```python
from build123d import *

# Parameters (mm, degrees)
SKETCH1_R           = 2
BOSS_EXTRUDE1_DEPTH = 16.85


with BuildPart() as part:
    # Sketch1 → Boss-Extrude1 (new body)
    # profile 1 of 4: a face of its own
    with BuildSketch(Plane(origin=(0, 0, 0), x_dir=(1, 0, 0), z_dir=(0, 1, 0))):
        Polygon((-24.645, 9), (-29.841152423, 0), (-24.841152423, 0), (0, 0), (0, 9), align=None)
        with Locations(Location((-14.92, 4.5, 0), (0, 0, 270))):
            Circle(SKETCH1_R, mode=Mode.SUBTRACT)
    # profile 2 of 4: a face of its own
    with BuildSketch(Plane(origin=(0, 0, 0), x_dir=(1, 0, 0), z_dir=(0, 1, 0))):
        Polygon((0, 9), (0, 0), (24.841152423, 0), (29.841152423, 0), (24.645, 9), align=None)
        with Locations(Location((14.92, 4.5, 0), (0, 0, 270))):
            Circle(SKETCH1_R, mode=Mode.SUBTRACT)
    # profile 3 of 4: a face of its own
    with BuildSketch(Plane(origin=(0, 0, 0), x_dir=(1, 0, 0), z_dir=(0, 1, 0))):
        with BuildLine():
            Line((-24.841152423, 0), (-29.841152423, 0))
            Line((-29.841152423, 0), (-42.542858345, -22))
            Line((-42.542858345, -22), (-38.697558883, -22))
            ThreePointArc((-38.697558883, -22), (-37.697558883, -21.732050808), (-36.965508076, -21))
            Line((-36.965508076, -21), (-24.841152423, 0))
        make_face()
    # profile 4 of 4: a face of its own
    with BuildSketch(Plane(origin=(0, 0, 0), x_dir=(1, 0, 0), z_dir=(0, 1, 0))):
        with BuildLine():
            Line((29.841152423, 0), (24.841152423, 0))
            Line((24.841152423, 0), (36.965508076, -21))
            ThreePointArc((36.965508076, -21), (37.697558883, -21.732050808), (38.697558883, -22))
            Line((38.697558883, -22), (42.542858345, -22))
            Line((42.542858345, -22), (29.841152423, 0))
        make_face()
    extrude(amount=BOSS_EXTRUDE1_DEPTH)


solid = part.part
```
Design review of the part built by this model. Coordinates are the model's own, in mm. A direction names the side the tool comes from. Round coordinates to 2 decimals unless told otherwise and drop trailing zeros. Order: outer loops, then holes, each group sorted by start corner. A loop starts at its lowest first (then second) coordinate and runs counter-clockwise, first axis right, second up. Notation, with made-up numbers: (41, 42.25) - (76, 42.25) arc R37 cw to (76, 78.25) - close; hole circle Ø1 at (57.5, 81). An arc over 180 degrees is marked (long way). One line per question, with ' | ' between items.
Item 1: Draft analysis for pull direction Z (two halves, no side actions). For faces 1 (the face through (0, 8, -9)), 2 (the face through (-16.872, 8.307, -4.934)), 3 (the face through (0, 0, -2)), 4 (the face through (0, 8, 0)), state which applies: +Z half, -Z half, draft (parallel to the pull), parting line (faces both ways), or undercut.
Checks:
face 1: -Z half | face 2: undercut | face 3: draft | face 4: +Z half
Item 2: For P1, Ø1.5, axis at x = -30.5, z = -0.5, coming from the -Y side; P2, Ø5, axis at x = -12, y = 6.5, coming from the +Z side; P3, Ø6, axis at y = 10, z = 16, coming from the -X side; P4, Ø1, axis at y = 13.5, z = 10.5, coming from the -X side, all flat-tipped, find the tip position at first contact; note any pin that passes through.
Checks:
P1: through | P2: z = 0 | P3: x = -40.81 | P4: x = -36.19
Item 3: Machinability: for faces 5 (the face through (15, 8.3, -6.5)), 6 (the face through (-30.99, 8.31, 10.65)), which of the approach directions +Z, -Z, +X, -X, +Y, -Y give a long, thin tool a straight path to every point of the face, cutting with its end or side? Answer none if there is none.
Checks:
face 5: +Y, -Y | face 6: +Z, +Y, -Y
Item 4: Take a section at D-D, the plane z = -4.5. Write out the cut boundary in (x, y), then the cut area to 3 significant figures.
Checks:
outline: (-27.24, 0) - (-16.92, 0) - (-16.92, 16.85) - (-27.24, 16.85) - close; (-12.92, 0) - (12.92, 0) - (12.92, 16.85) - (-12.92, 16.85) - close; (16.92, 0) - (27.24, 0) - (27.24, 16.85) - (16.92, 16.85) - close | area: 783 mm²
Item 5: Wall thickness on line 1 (Z direction, x = 6.5, y = 2.5); line 2 (X direction, y = 12.25, z = -4.5); line 3 (X direction, y = 6.25, z = 1): over which ranges is each line inside the solid? List them lowest first. Write a range as [from, to].
Checks:
line 1: [-9, 0] | line 2: [-27.24, -16.92], [-12.92, 12.92], [16.92, 27.24] | line 3: [-30.42, -25.42], [25.42, 30.42]
Item 6: Take a section at A-A, the plane x = 14.92. Write out the cut boundary in (y, z), then the cut area to 4 significant figures.
Checks:
outline: (0, -9) - (16.85, -9) - (16.85, -6.5) - (0, -6.5) - close; (0, -2.5) - (16.85, -2.5) - (16.85, 0) - (0, 0) - close | area: 84.25 mm²
Item 7: Take a section at C-C, the plane z = 16.5. Write out the cut boundary in (x, y).
Checks:
outline: (-39.37, 0) - (-34.37, 0) - (-34.37, 16.85) - (-39.37, 16.85) - close; (34.37, 0) - (39.37, 0) - (39.37, 16.85) - (34.37, 16.85) - close
Item 8: Take a section at B-B, the plane y = 5.5. Write out the cut boundary in (x, z) (1 decimal).
Checks:
outline: (-42.5, 22) - (-24.6, -9) - (24.6, -9) - (42.5, 22) - (38.7, 22) arc R2 ccw to (37, 21) - (24.8, 0) - (-24.8, 0) - (-37, 21) arc R2 ccw to (-38.7, 22) - close; hole circle Ø4 at (-14.9, -4.5); hole circle Ø4 at (14.9, -4.5)
